Could you check a few things on this model? Use its own coordinates, in mm. Face numbers are marked on the shaded views. A direction names the side the tool comes from. Coordinates: 2 decimals unless noted, no trailing zeros. Order: outer loops, then holes, each group sorted by start corner. A loop starts at its lowest first (then second) coordinate and runs counter-clockwise, first axis right, second up. Notation, with made-up numbers: (7.25, 62) -> (29.25, 62) arc R20 ccw to (29.25, 97) -> close; hole circle Ø10 at (84, -39). An arc over 180 degrees is marked (long way). Use a Markdown table: item, result. Add a question column.
1) If I drill on L1, parallel to X at y = 0.3, z = 120.65 (1 decimal); L2, parallel to X at y = 1.25, z = 14, over which ranges is the centre line in solid material (lowest first)? Write a range as [from, to].
2) If we section it at B-B (x = 8): Write out the boundary of the cut face in (y, z).
3) Which directions (+Z, -Z, +X, -X, +Y, -Y) give clear straight access to the entire face, cutting with the end or side of a thin tool? Please do the marked faces 1 and 2.
4) If we section it at A-A (z = 120.65): Write out the boundary of the cut face in (x, y) (1 decimal), plus the area to 3 significant figures.
5) If we section it at C-C (z = 71.5): Write out the boundary of the cut face in (x, y) (3 decimals), plus the area to 3 significant figures.
6) Will these pins go through, and if not, where does the flat tip stop? pin 1 Ø3 at (x, y) = (2, 7) entering from +Z; pin 2 Ø6 at (x, z) = (7.94, 120.65) entering from +Y.
7) If we section it at D-D (y = 4): Write out the boundary of the cut face in (x, z).
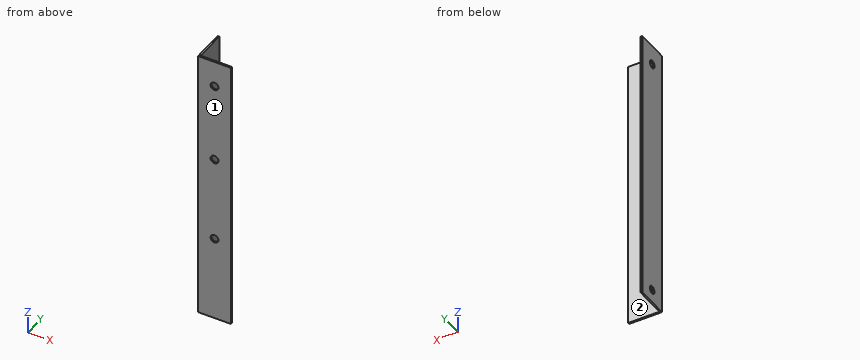
Autodesk Inventor part; units mm, degrees
ref_plane "YZ Plane" through (0, 0, 0) normal (1, 0, 0) x (0, 1, 0)
ref_plane "XZ Plane" through (0, 0, 0) normal (0, 1, 0) x (-1, 0, 0)
ref_plane "XY Plane" through (0, 0, 0) normal (0, 0, 1) x (1, 0, 0)
sketch "Sketch1" plane through (0, 0, 0) normal (0, 0, 1) x (1, 0, 0)
  line L0 (0, 0) -> (0, 15.875)
  line L1 (0, 15.875) -> (0.7937, 15.875)
  line L2 (0.7937, 15.875) -> (0.7938, 0.7937)
  line L3 (0.7938, 0.7937) -> (15.875, 0.7937)
  line L4 (15.875, 0.7937) -> (15.875, 0)
  line L5 (15.875, 0) -> (0, 0)
  dimension "d0" = 15.875
  dimension "d1" = 0.7937
extrude "Extrusion1" add sketch "Sketch1" along normal blind 133.35
sketch "Sketch2" plane through (0, 0, 0) normal (0, -1, 0) x (1, 0, 0)
  line L0 (15.875, 0) -> (0, 0)
  line L1 (0, 133.35) -> (15.875, 133.35)
  line L2 (7.9375, 133.35) -> (7.9375, 0) construction
  circle A0 centre (7.9375, 120.65) radius 1.905
  circle A1 centre (7.9375, 41.275) radius 1.905
  circle A2 centre (7.9375, 82.55) radius 1.905
  dimension "d4" = 3.81
  dimension "d6" = 12.7
  dimension "d7" = 41.275
  dimension "d16" = 38.1
extrude "Extrusion2" cut sketch "Sketch2" against normal through all
sketch "Sketch3" plane through (0, 0, 0) normal (-1, 0, 0) x (0, 0, 1)
  line L0 (0, 0) -> (0, 15.875)
  line L1 (133.35, 15.875) -> (133.35, 0)
  line L2 (0, 7.9375) -> (133.35, 7.9375) construction
  circle A0 centre (6.35, 7.9375) radius 1.905
  circle A1 centre (123.825, 7.9375) radius 1.905
  dimension "d11" = 3.81
  dimension "d12" = 9.525
  dimension "d13" = 6.35
extrude "Extrusion3" cut sketch "Sketch3" against normal through all
properties part number "Hopper Bracing P3" material "Aluminum 6061"
Answer sheet:
| question | item | result |
|---|---|---|
| 1 | L1 | [0, 6], [9.8, 15.9] |
| 1 | L2 | [0, 0.79] |
| 2 | outline | (0, 0) -> (0.79, 0) -> (0.79, 39.37) -> (0, 39.37) -> close; (0, 43.18) -> (0.79, 43.18) -> (0.79, 80.65) -> (0, 80.65) -> close; (0, 84.45) -> (0.79, 84.45) -> (0.79, 118.75) -> (0, 118.75) -> close; (0, 122.55) -> (0.79, 122.55) -> (0.79, 133.35) -> (0, 133.35) -> close |
| 3 | face 1 | +Z, -Z, +X, -X, -Y |
| 3 | face 2 | +Z, -Z, +X, +Y |
| 4 | outline | (0, 0) -> (6, 0) -> (6, 0.8) -> (0.8, 0.8) -> (0.8, 15.9) -> (0, 15.9) -> close; (9.8, 0) -> (15.9, 0) -> (15.9, 0.8) -> (9.8, 0.8) -> close |
| 4 | area | 21.5 mm2 |
| 5 | outline | (0, 0) -> (15.875, 0) -> (15.875, 0.794) -> (0.794, 0.794) -> (0.794, 15.875) -> (0, 15.875) -> close |
| 5 | area | 24.6 mm2 |
| 6 | pin 1 | z = 133.35 |
| 6 | pin 2 | y = 0.79 |
| 7 | outline | (0, 0) -> (0.79, 0) -> (0.79, 133.35) -> (0, 133.35) -> close |
